The model under review builds one solid part; all positions refer to its coordinate system, in mm. Coordinates: 2 decimals unless noted, no trailing zeros. Write each loop counter-clockwise with the first axis right and the second up, starting at its lowest first coordinate (ties: lowest second). Pieces come first, ordered by that corner, then holes.
1) For line 1 (Z direction, x = 322, y = 6); line 2 (Y direction, x = 370.5, z = -127), list the stretches that pass through material, from the lowest coordinate up.
2) Add section A-A, the plane y = 3.75. State the section outline as (x, z) points, then the cut area to 3 significant figures.
3) For P1, Ø6.5, axis at x = 170, z = -120, coming from the +Y side, flat-tipped, find the tip position at first contact; note if it passes through.
4) Add section B-B, the plane x = 316.5. State the section outline as (y, z) points.
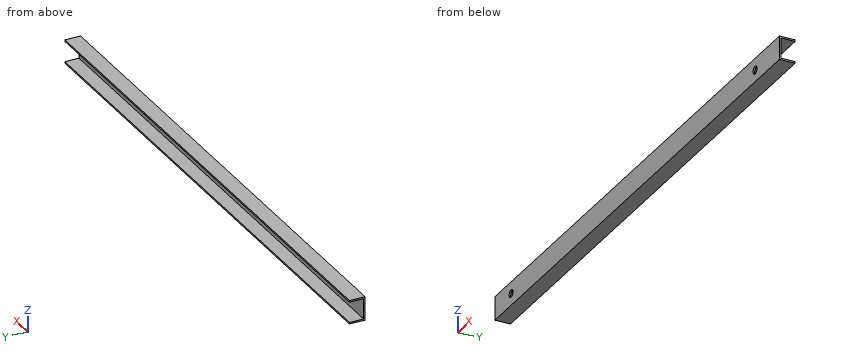
from build123d import *

# Parameters (mm, degrees)
SKETCH2_W           = 350
SKETCH2_H           = 15
BOSS_EXTRUDE1_DEPTH = 10
SKETCH3_W           = 350
SKETCH3_H           = 13
CUT_EXTRUDE1_DEPTH  = 9
SKETCH4_R           = 2.4
SKETCH4_R_2         = 2.5
CUT_EXTRUDE3_DEPTH  = 10


with BuildPart() as part:
    # Sketch2 → Boss-Extrude1 (new body)
    with BuildSketch(Plane(origin=(0, 0, 0), x_dir=(1, 0, 0), z_dir=(0, 1, 0))):
        with Locations((214.483557787, 122.439976597)):
            Rectangle(SKETCH2_W, SKETCH2_H)
    extrude(amount=BOSS_EXTRUDE1_DEPTH)

    # Sketch3 → Cut-Extrude1 (cut)
    with BuildSketch(Plane(origin=(0, 10, 0), x_dir=(1, 0, 0), z_dir=(0, 1, 0))):
        with Locations((214.483557787, 122.439976597)):
            Rectangle(SKETCH3_W, SKETCH3_H)
    extrude(amount=-CUT_EXTRUDE1_DEPTH, mode=Mode.SUBTRACT)

    # Sketch4 → Cut-Extrude3 (cut)
    with BuildSketch(Plane(origin=(0, 1, 0), x_dir=(1, 0, 0), z_dir=(0, 1, 0))):
        with Locations((59.483557787, 122.439976597)):
            Circle(SKETCH4_R)
        with Locations((359.483557787, 122.439976597)):
            Circle(SKETCH4_R_2)
    extrude(amount=-CUT_EXTRUDE3_DEPTH, mode=Mode.SUBTRACT)


solid = part.part
Geometry results:
1. line 1: z = -129.94 to -128.94, -115.94 to -114.94
1. line 2: y = 0 to 1
2. outline: (39.48, -129.94) - (389.48, -129.94) - (389.48, -128.94) - (39.48, -128.94) - close; (39.48, -115.94) - (389.48, -115.94) - (389.48, -114.94) - (39.48, -114.94) - close
2. area: 700 mm2
3. P1: stops at y = 1
4. outline: (0, -129.94) - (10, -129.94) - (10, -128.94) - (1, -128.94) - (1, -115.94) - (10, -115.94) - (10, -114.94) - (0, -114.94) - close
